```python
from build123d import *

# Parameters (mm, degrees)
CROQUIS1_W              = 120
CROQUIS1_H              = 90
SALIENTE_EXTRUIR1_DEPTH = 100
CROQUIS2_W              = 115
CROQUIS2_H              = 85
CORTAR_EXTRUIR1_DEPTH   = 97.5
CROQUIS3_W              = 60
CROQUIS3_H              = 90
CROQUIS3_W_2            = 120
CROQUIS3_H_2            = 45
CROQUIS3_W_3            = 115
CROQUIS3_H_3            = 85
SALIENTE_EXTRUIR2_DEPTH = 2.5


with BuildPart() as part:
    # Croquis1 → Saliente-Extruir1 (new body)
    with BuildSketch(Plane.XY):
        Rectangle(CROQUIS1_W, CROQUIS1_H)
    extrude(amount=SALIENTE_EXTRUIR1_DEPTH)

    # Croquis2 → Cortar-Extruir1 (cut)
    with BuildSketch(Plane(origin=(0, 0, 0), x_dir=(-1, 0, 0), z_dir=(0, 0, -1))):
        Rectangle(CROQUIS2_W, CROQUIS2_H)
    extrude(amount=-CORTAR_EXTRUIR1_DEPTH, mode=Mode.SUBTRACT)

    # Croquis3 → Saliente-Extruir2 (add)
    # profile 1 of 5: a face of its own
    with BuildSketch(Plane(origin=(0, 0, 0), x_dir=(-1, 0, 0), z_dir=(0, 0, -1))):
        with Locations((-90, 0)):
            Rectangle(CROQUIS3_W, CROQUIS3_H)
    # profile 2 of 5: a face of its own
    with BuildSketch(Plane(origin=(0, 0, 0), x_dir=(-1, 0, 0), z_dir=(0, 0, -1))):
        with Locations((0, 67.5)):
            Rectangle(CROQUIS3_W_2, CROQUIS3_H_2)
    # profile 3 of 5: a face of its own
    with BuildSketch(Plane(origin=(0, 0, 0), x_dir=(-1, 0, 0), z_dir=(0, 0, -1))):
        Rectangle(CROQUIS3_W_2, CROQUIS3_H)
        Rectangle(CROQUIS3_W_3, CROQUIS3_H_3, mode=Mode.SUBTRACT)
    # profile 4 of 5: a face of its own
    with BuildSketch(Plane(origin=(0, 0, 0), x_dir=(-1, 0, 0), z_dir=(0, 0, -1))):
        with Locations((90, 0)):
            Rectangle(CROQUIS3_W, CROQUIS3_H)
    # profile 5 of 5: a face of its own
    with BuildSketch(Plane(origin=(0, 0, 0), x_dir=(-1, 0, 0), z_dir=(0, 0, -1))):
        with Locations((0, -67.5)):
            Rectangle(CROQUIS3_W_2, CROQUIS3_H_2)
    extrude(amount=-SALIENTE_EXTRUIR2_DEPTH)


solid = part.part
```
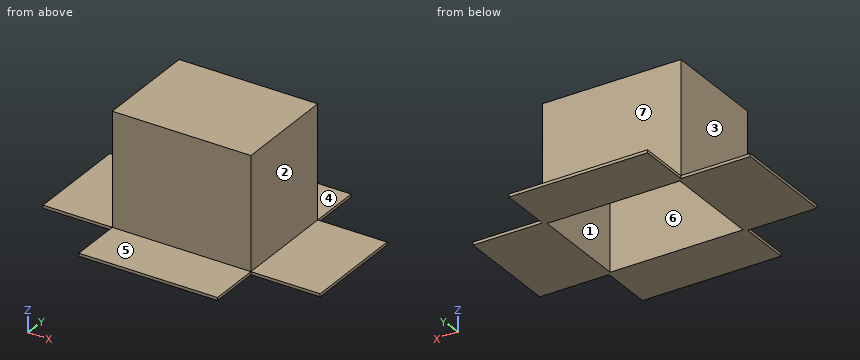
Here's how the part is built. I have some questions about the finished solid (model axes, mm). Face numbers are marked on the shaded views. A direction names the side the tool comes from. Round coordinates to 2 decimals unless told otherwise and drop trailing zeros. Order: outer loops, then holes, each group sorted by start corner. A loop starts at its lowest first (then second) coordinate and runs counter-clockwise, first axis right, second up. Notation, with made-up numbers: M -22,57 L 34,57 A21 ccw 34,65 Z; hole C 0,38.5 d6. An arc over 180 degrees is marked long. Answer as CSV lines item,"result".
Item 1: For pin 1 (8 mm diameter, centred on y = -8, z = 37.5, fed in from +X); pin 2 (0.8 mm diameter, centred on x = 95.5, z = 1, fed in from -Y); pin 3 (1 mm diameter, centred on x = 21, y = -15.5, fed in from -Z); pin 4 (8 mm diameter, centred on y = -52.5, z = 27, fed in from -X), each with a flat end and sliding along its axis, tell me the tip position at first contact or that it passes through.
From the geometry:
pin 1,"x = 60"
pin 2,"y = -45"
pin 3,"z = 97.5"
pin 4,"through"
Item 2: Which directions (+Z, -Z, +X, -X, +Y, -Y) give clear straight access to the entire face, cutting with the end or side of a thin tool? Please do the marked faces 5, 6 and 7.
From the geometry:
face 5,"+Z, +X, -X, -Y"
face 6,"-Z"
face 7,"+Z, +X, -X, +Y"
Item 3: Please list where these lines run through material, in increasing order: L1, parallel to Y at x = 0, z = 22.5; L2, parallel to X at y = -16.5, z = 37.5; L3, parallel to Z at x = 105, y = -22. Write a range as [from, to].
From the geometry:
L1,"[-45, -42.5], [42.5, 45]"
L2,"[-60, -57.5], [57.5, 60]"
L3,"[0, 2.5]"
Item 4: Imagine slicing it at D-D on x = -83. List the corners of the cut face in (y, z) for me.
From the geometry:
outline,"M -45,0 L 45,0 L 45,2.5 L -45,2.5 Z"
Item 5: We'd pull the mould along X, two halves only. Please class the marked faces 1, 2, 3 and 4: +X half, -X half, draft (parallel to the pull), parting line (faces both ways), or undercut.
From the geometry:
face 1,"undercut"
face 2,"+X half"
face 3,"-X half"
face 4,"draft"
Item 6: Imagine slicing it at A-A on z = 6. List the corners of the cut face in (x, y) for me, and give its area (4 significant figures).
From the geometry:
outline,"M -60,-45 L 60,-45 L 60,45 L -60,45 Z; hole M -57.5,-42.5 L 57.5,-42.5 L 57.5,42.5 L -57.5,42.5 Z"
area,"1,025 mm2"
Item 7: Imagine slicing it at C-C on y = 53. List the corners of the cut face in (x, z) for me, and give its area (3 significant figures).
From the geometry:
outline,"M -60,0 L 60,0 L 60,2.5 L -60,2.5 Z"
area,"300 mm2"
Item 8: Imagine slicing it at B-B on x = 43.5. List the corners of the cut face in (y, z) for me.
From the geometry:
outline,"M -90,0 L -42.5,0 L -42.5,97.5 L 42.5,97.5 L 42.5,0 L 90,0 L 90,2.5 L 45,2.5 L 45,100 L -45,100 L -45,2.5 L -90,2.5 Z"
